The drawing under review shows one solid part. Ordinate dimensions are in mm from its lowest x, y, z. A direction names the side the tool comes from. Give positions to 0.01 mm unless a question says otherwise; leave off trailing zeros. Order: outer loops, then holes, each group sorted by start corner. A loop starts at its lowest first (then second) coordinate and runs counter-clockwise, first axis right, second up. Notation, with made-up numbers: (70.25, -5.5) -> (121.25, -5.5) arc R24 ccw to (121.25, 8.5) -> close; hole circle Ø8 at (-30, 12.5). An arc over 180 degrees is marked (long way). Use CSV: the item, a comma, the result in double quotes. Start each with the question number.
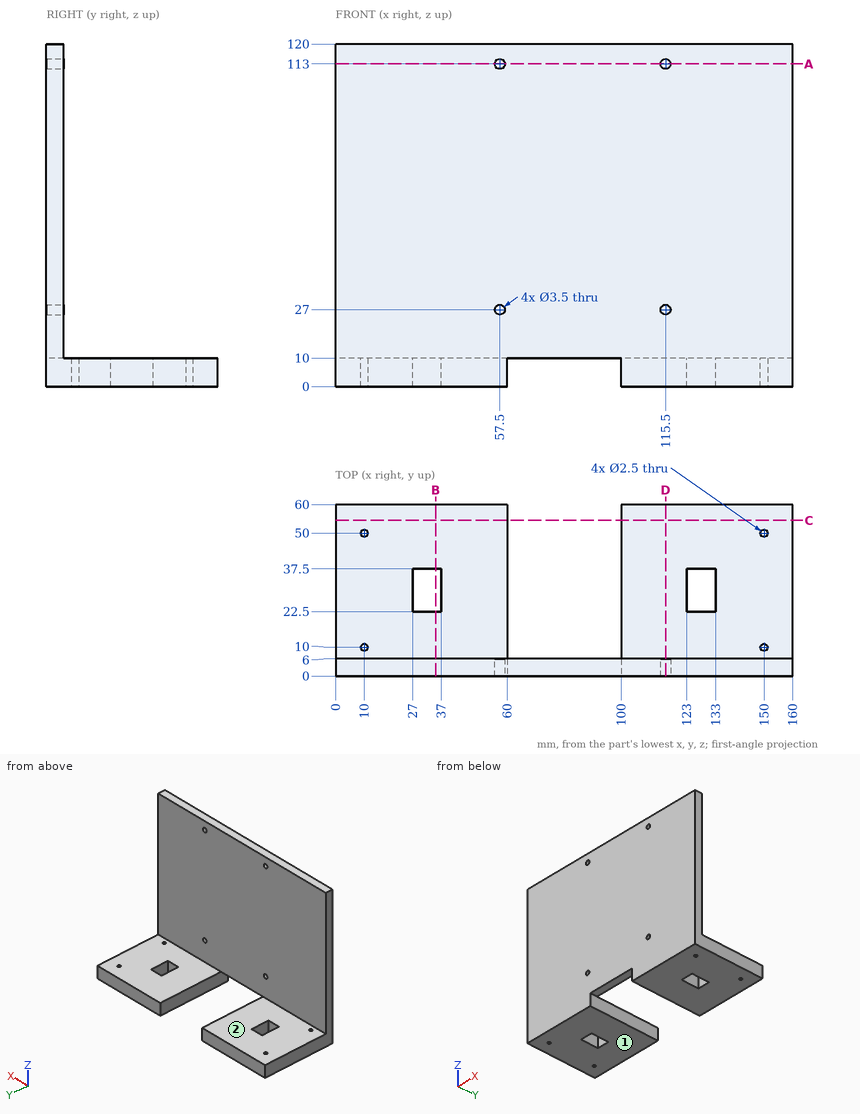
1. For the marked faces 1 and 2, list the 3-axis set-ups (+Z, -Z, +X, -X, +Y, -Y) from which the entire face can be reached by the end or side of a thin tool; tool diameter is ignored.
2. Consider section C-C (y = 54.5). State the section outline as (x, z) points.
3. Consider section D-D (x = 115.5). State the section outline as (y, z) points, plus the area to 3 significant figures.
4. Consider section B-B (x = 35). State the section outline as (y, z) points, plus the area to 3 significant figures.
5. To check wall thickness, follow L1, parallel to X at y = 4.75, z = 113; L2, parallel to Y at x = 10, z = 6; L3, parallel to Z at x = 115.5, y = 2.35. State the ranges of each line that lie inside material, in increasing order. Write a range as [from, to].
6. Clearance check with flat-ended pins moving along their axes: P1, Ø2, axis at x = 37, y = 31.5, coming from the +Z side; P2, Ø1.5, axis at x = 150, y = 10, coming from the +Z side; P3, Ø6, axis at x = 139, z = 105.5, coming from the +Y side. State where each tip first meets the part, or that it passes through.
7. Consider section A-A (z = 113). State the section outline as (x, y) points.
Answer list:
1,face 1,"-Z, +X, -X, +Y, -Y"
1,face 2,"+Z, +X, -X, +Y"
2,outline,"(0, 0) -> (60, 0) -> (60, 10) -> (0, 10) -> close; (100, 0) -> (160, 0) -> (160, 10) -> (100, 10) -> close"
3,outline,"(0, 0) -> (60, 0) -> (60, 10) -> (6, 10) -> (6, 25.25) -> (0, 25.25) -> close; (0, 28.75) -> (6, 28.75) -> (6, 111.25) -> (0, 111.25) -> close; (0, 114.75) -> (6, 114.75) -> (6, 120) -> (0, 120) -> close"
3,area,"1,220 mm2"
4,outline,"(0, 0) -> (22.5, 0) -> (22.5, 10) -> (6, 10) -> (6, 120) -> (0, 120) -> close; (37.5, 0) -> (60, 0) -> (60, 10) -> (37.5, 10) -> close"
4,area,"1,110 mm2"
5,L1,"[0, 55.75], [59.25, 113.75], [117.25, 160]"
5,L2,"[0, 8.75], [11.25, 48.75], [51.25, 60]"
5,L3,"[0, 25.25], [28.75, 111.25], [114.75, 120]"
6,P1,"z = 10"
6,P2,"through"
6,P3,"y = 6"
7,outline,"(0, 0) -> (55.75, 0) -> (55.75, 6) -> (0, 6) -> close; (59.25, 0) -> (113.75, 0) -> (113.75, 6) -> (59.25, 6) -> close; (117.25, 0) -> (160, 0) -> (160, 6) -> (117.25, 6) -> close"
